Part print with two shaded views. Sizes in mm from the minimum x, y, z corner. Give positions to 0.01 mm unless a question says otherwise; leave off trailing zeros. Order: outer loops, then holes, each group sorted by start corner. A loop starts at its lowest first (then second) coordinate and runs counter-clockwise, first axis right, second up.
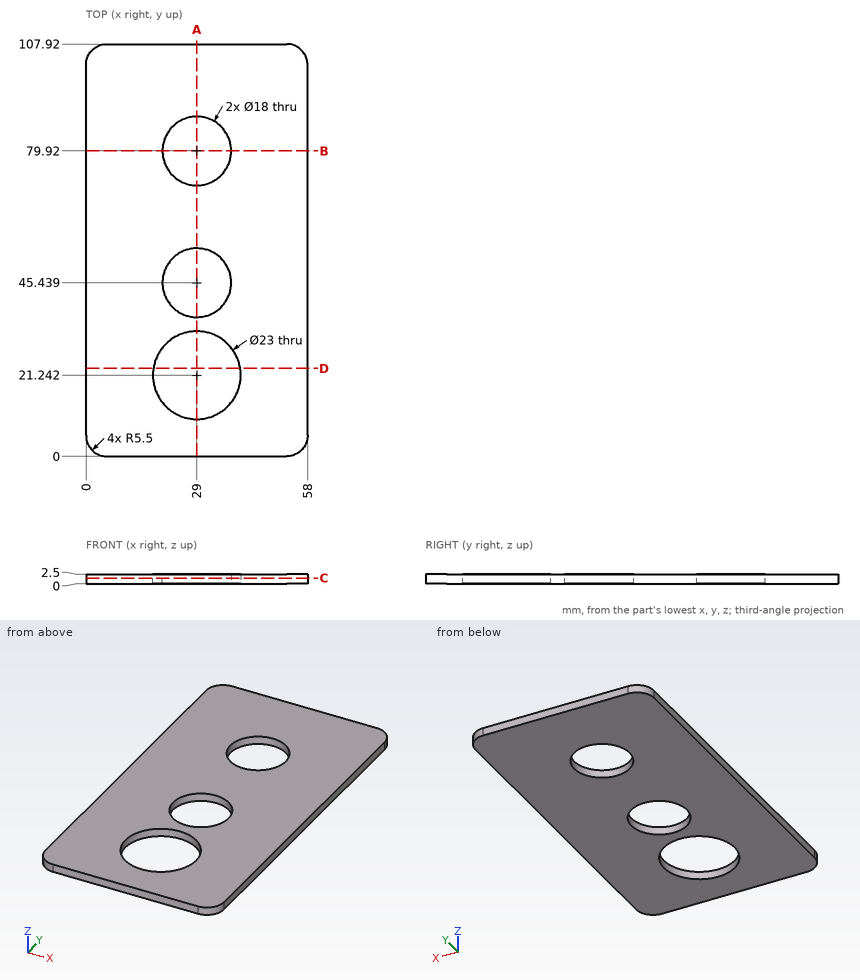
Item 1: Slice it at B-B (y = 79.92). Give the cut face in (x, z).
Item 2: Slice it at A-A (x = 29). Give the cut face in (y, z).
Item 3: Drop a flat-ended pin along its axis: pin 1 Ø11 at (x, y) = (29, 45.44) entering from +Z. Give the stop position or say it passes through.
Item 4: Wall check: L1, parallel to Y at x = 29, z = 1.1; L2, parallel to Y at x = 32, z = 0.65 (1 decimal); L3, parallel to Y at x = 53, z = 0.35. Give the ranges that are in metal, low to high.
Item 5: Slice it at C-C (z = 1.55). Give the cut face in (x, y).
Item 6: Slice it at D-D (y = 23). Give the cut face in (x, z) (1 decimal).
A:
1. outline: (0, 0) - (20, 0) - (20, 2.5) - (0, 2.5) - close; (38, 0) - (58, 0) - (58, 2.5) - (38, 2.5) - close
2. outline: (0, 0) - (9.74, 0) - (9.74, 2.5) - (0, 2.5) - close; (32.74, 0) - (36.44, 0) - (36.44, 2.5) - (32.74, 2.5) - close; (54.44, 0) - (70.92, 0) - (70.92, 2.5) - (54.44, 2.5) - close; (88.92, 0) - (107.92, 0) - (107.92, 2.5) - (88.92, 2.5) - close
3. pin 1: passes through
4. L1: y = 0 to 9.74, 32.74 to 36.44, 54.44 to 70.92, 88.92 to 107.92
4. L2: y = 0 to 10.1, 32.3 to 37, 53.9 to 71.4, 88.4 to 107.9
4. L3: y = 0.02 to 107.9
5. outline: (0, 5.5) arc R5.5 ccw to (5.5, 0) - (52.5, 0) arc R5.5 ccw to (58, 5.5) - (58, 102.42) arc R5.5 ccw to (52.5, 107.92) - (5.5, 107.92) arc R5.5 ccw to (0, 102.42) - close; hole circle Ø23 at (29, 21.24); hole circle Ø18 at (29, 45.44); hole circle Ø18 at (29, 79.92)
6. outline: (0, 0) - (17.6, 0) - (17.6, 2.5) - (0, 2.5) - close; (40.4, 0) - (58, 0) - (58, 2.5) - (40.4, 2.5) - close
